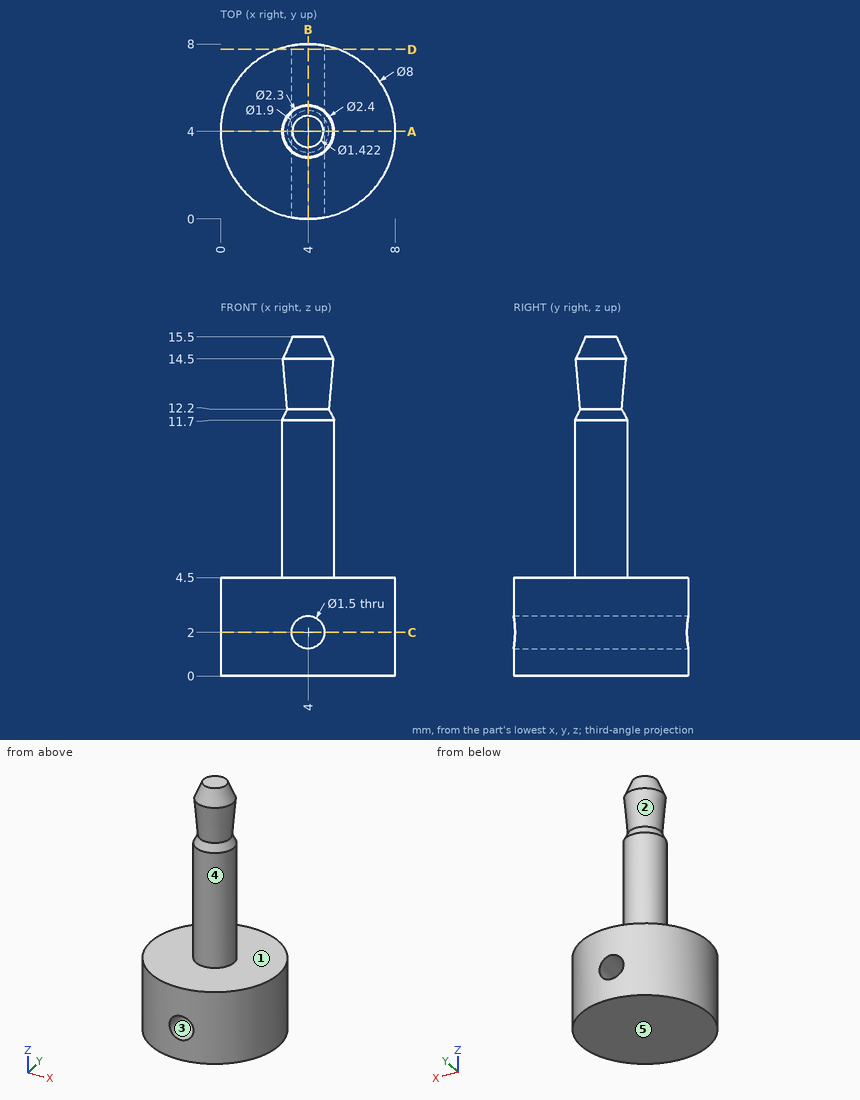
Verification items for this drawing (mm, ordinates from the low corner). A direction names the side the tool comes from. Give positions to 0.01 mm unless a question says otherwise; leave off trailing zeros. Write each loop counter-clockwise with the first axis right and the second up, starting at its lowest first coordinate (ties: lowest second). Pieces come first, ordered by that corner, then holes. Notation, with made-up numbers: (37.5, 16) - (45.5, 16) arc R21 cw to (45.5, 50) - close; hole circle Ø10 at (8, -38). An arc over 180 degrees is marked (long way). Answer as a JSON object with one key per item and string values. Group by question number.
1) Thickness scan on probe 1 along Z at (x, y) = (4, 2.25); probe 2 along Z at (x, y) = (5.25, 1.75); probe 3 along X at (y, z) = (4.75, 2.25). Record the ranges inside material, lowest first. Write a range as from..to.
2) Sectioned sample at A-A (y = 4). Record the cut outline in (x, z).
3) Sectioned sample at C-C (z = 2). Record the cut outline in (x, y).
4) Sectioned sample at D-D (y = 7.75). Record the cut outline in (x, z).
5) Depth check by flat-ended pin: P1, Ø0.9, axis at x = 4, z = 2, coming from the -Y side; P2, Ø3, axis at y = 4, z = 10, coming from the -X side; P3, Ø2, axis at x = 1, z = 2, coming from the -Y side (1 decimal). Enter the tip coordinate at first touch or a pass-through.
6) Access from +Z, -Z, +X, -X, +Y, -Y to the whole of each face (thin tool, end or side, straight path). Record for the marked faces 4 and 5.
7) Release check for a two-part mould opening along X. For the marked faces 1, 2 and 3 record: pulls with the +X half, pulls with the -X half, needs draft (parallel to the pull), parting line crosses it, or undercut.
8) Sectioned sample at B-B (x = 4). Record the cut outline in (y, z).
Geometry results:
{
 "1": {"probe 1": "z = 0..1.25, 2.75..4.5", "probe 2": "z = 0..4.5", "probe 3": "x = 0.07..3.29, 4.71..7.93"},
 "2": {"outline": "(0, 0) - (8, 0) - (8, 4.5) - (5.2, 4.5) - (5.2, 11.7) - (4.95, 12.2) - (5.15, 14.5) - (4.71, 15.5) - (3.29, 15.5) - (2.85, 14.5) - (3.05, 12.2) - (2.8, 11.7) - (2.8, 4.5) - (0, 4.5) - close; hole circle Ø1.5 at (4, 2)"},
 "3": {"outline": "(3.25, 0.07) - (3.25, 7.93) arc R4 ccw to start; (4.75, 0.07) arc R4 ccw to (4.75, 7.93) - close"},
 "4": {"outline": "(2.61, 0) - (5.39, 0) - (5.39, 4.5) - (2.61, 4.5) - close; hole circle Ø1.5 at (4, 2)"},
 "5": {"P1": "passes through", "P2": "stops at x = 2.8", "P3": "stops at y = 0.5"},
 "6": {"face 4": "+Z", "face 5": "-Z, +X, -X, +Y, -Y"},
 "7": {"face 1": "needs draft", "face 2": "parting line crosses it", "face 3": "undercut"},
 "8": {"outline": "(0, 0) - (8, 0) - (8, 1.25) - (0, 1.25) - close; (0, 2.75) - (8, 2.75) - (8, 4.5) - (5.2, 4.5) - (5.2, 11.7) - (4.95, 12.2) - (5.15, 14.5) - (4.71, 15.5) - (3.29, 15.5) - (2.85, 14.5) - (3.05, 12.2) - (2.8, 11.7) - (2.8, 4.5) - (0, 4.5) - close"}
}
